```python
from build123d import *

# Parameters (mm, degrees)
SKETCH1_W           = 15
SKETCH1_H           = 5
BOSS_EXTRUDE1_DEPTH = 2.5


with BuildPart() as part:
    # Sketch1 → Boss-Extrude1 (new, symmetric)
    with BuildSketch(Plane.XY):
        Polygon((430, 300), (430, 255), (422.5, 255), (422.5, 245), (407.5, 245), (407.5, 255), (400, 255), (400, 430), (407.5, 430), (407.5, 440), (422.5, 440), (422.5, 430), (430, 430), (430, 385), (435, 385), (435, 370), (430, 370), (430, 350), (435, 350), (435, 335), (430, 335), (430, 315), (435, 315), (435, 300), align=None)
        with Locations((412.5, 402.5)):
            Rectangle(SKETCH1_W, SKETCH1_H, mode=Mode.SUBTRACT)
    extrude(amount=BOSS_EXTRUDE1_DEPTH, both=True)


solid = part.part
```
Check sheet for the modelled part. Datum: model origin and axes. Units: mm. A direction names the side the tool comes from. Round coordinates to 2 decimals unless told otherwise and drop trailing zeros. Write each loop counter-clockwise with the first axis right and the second up, starting at its lowest first coordinate (ties: lowest second). Pieces come first, ordered by that corner, then holes. Notation, with made-up numbers: (66.25, 33.25) -> (84.25, 33.25) arc R28 cw to (84.25, 65.25) -> close; hole circle Ø5 at (13.25, -18.5). An arc over 180 degrees is marked (long way). One line per question, with ' | ' between items. Start each with the question number.
1. Set-up check for faces 4 (the face through (426, 255, 0)), 5 (the face through (430, 408, 0)), 6 (the face through (430, 360, 0)), 7 (the face through (407.5, 435, 0)), 8 (the face through (412, 405, 0)): record each of +Z, -Z, +X, -X, +Y, -Y from which the full face is reachable in a straight line by a thin tool's end or side.
2. Scan lines: line 1 along Y through (x, z) = (405.5, -1.6); line 2 along Y through (x, z) = (411, 2.3); line 3 along Y through (x, z) = (427.5, 2.15). Record each from-to range of solid material in increasing order. Write a range as from..to.
3. Sectioned sample at A-A, the plane x = 432.5. Record the cut outline in (y, z).
4. Sectioned sample at D-D, the plane y = 279.5. Record the cut outline in (x, z).
5. Depth check by flat-ended pin: pin 1 (3 mm diameter, centred on x = 429.5, z = 0, fed in from -Y); pin 2 (1.5 mm diameter, centred on x = 431.5, z = -0.5, fed in from -Y); pin 3 (1.5 mm diameter, centred on x = 432, z = 1, fed in from +Y). Enter the tip coordinate at first touch or a pass-through.
6. Sectioned sample at B-B, the plane z = -0.8. Record the cut outline in (x, y), then the cut area to 3 significant figures.
7. Release check for a two-part mould opening along X. For faces 1 (the face through (426, 430, 0)), 2 (the face through (407.5, 250, 0)), 3 (the face through (405, 402, 0)) record: +X half, -X half, draft (parallel to the pull), parting line (faces both ways), or undercut.
8. Sectioned sample at C-C, the plane x = 410. Record the cut outline in (y, z), then the cut area to 3 significant figures.
Taken from the geometry:
1) face 4: +Z, -Z, +X, -Y | face 5: +Z, -Z, +X, +Y | face 6: +Z, -Z, +X | face 7: +Z, -Z, -X, +Y | face 8: +Z, -Z
2) line 1: y = 255..400, 405..430 | line 2: y = 245..400, 405..440 | line 3: y = 255..430
3) outline: (300, -2.5) -> (315, -2.5) -> (315, 2.5) -> (300, 2.5) -> close; (335, -2.5) -> (350, -2.5) -> (350, 2.5) -> (335, 2.5) -> close; (370, -2.5) -> (385, -2.5) -> (385, 2.5) -> (370, 2.5) -> close
4) outline: (400, -2.5) -> (430, -2.5) -> (430, 2.5) -> (400, 2.5) -> close
5) pin 1: stops at y = 255 | pin 2: stops at y = 300 | pin 3: stops at y = 385
6) outline: (400, 255) -> (407.5, 255) -> (407.5, 245) -> (422.5, 245) -> (422.5, 255) -> (430, 255) -> (430, 300) -> (435, 300) -> (435, 315) -> (430, 315) -> (430, 335) -> (435, 335) -> (435, 350) -> (430, 350) -> (430, 370) -> (435, 370) -> (435, 385) -> (430, 385) -> (430, 430) -> (422.5, 430) -> (422.5, 440) -> (407.5, 440) -> (407.5, 430) -> (400, 430) -> close; hole (405, 400) -> (420, 400) -> (420, 405) -> (405, 405) -> close | area: 5,700 mm^2
7) face 1: draft | face 2: -X half | face 3: undercut
8) outline: (245, -2.5) -> (400, -2.5) -> (400, 2.5) -> (245, 2.5) -> close; (405, -2.5) -> (440, -2.5) -> (440, 2.5) -> (405, 2.5) -> close | area: 950 mm^2
